The drawing under review shows one solid part. Ordinate dimensions are in mm from its lowest x, y, z. Round coordinates to 2 decimals unless told otherwise and drop trailing zeros. Order: outer loops, then holes, each group sorted by start corner. A loop starts at its lowest first (then second) coordinate and runs counter-clockwise, first axis right, second up. Notation, with made-up numbers: M -39.75,36 L 19.25,36 A12 ccw 19.25,48 Z; hole C -9,-5.5 d4. An arc over 180 degrees is marked long. Answer as a JSON object with one key per item and string values. Group by question number.
1. Clearance check with flat-ended pins moving along their axes: P1, Ø6, axis at x = 23, y = 5, coming from the -Z side; P2, Ø3.5, axis at x = 50, y = 12.5, coming from the -Z side. State where each tip first meets the part, or that it passes through.
2. To check wall thickness, follow probe 1 along Y at (x, z) = (50, 3.5); probe 2 along X at (y, z) = (12.5, 4.25); probe 3 along X at (y, z) = (13.25, 0.5). State the ranges of each line that lie inside material, in increasing order. Write a range as [from, to].
3. Add section B-B on y = 12.5. State the section outline as (x, z) points, and give its area (3 significant figures).
4. Add section A-A on x = 50. State the section outline as (y, z) points, and give its area (3 significant figures).
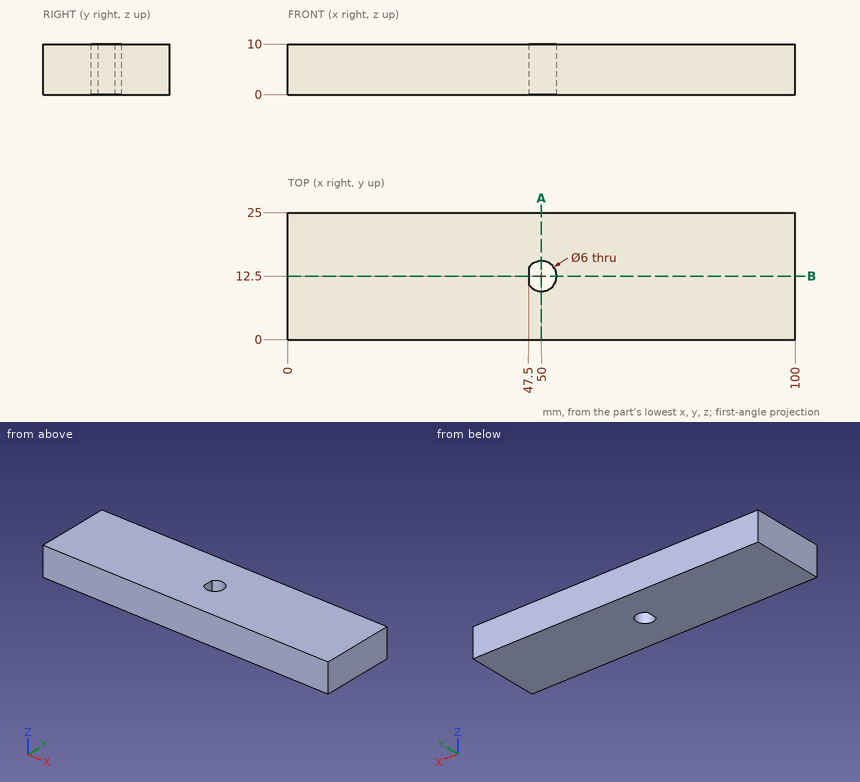
Recorded:
{
 "1": {"P1": "stops at z = 0", "P2": "passes through"},
 "2": {"probe 1": "y = [0, 9.5], [15.5, 25]", "probe 2": "x = [0, 47.5], [53, 100]", "probe 3": "x = [0, 47.5], [52.9, 100]"},
 "3": {"outline": "M 0,0 L 47.5,0 L 47.5,10 L 0,10 Z; M 53,0 L 100,0 L 100,10 L 53,10 Z", "area": "945 mm²"},
 "4": {"outline": "M 0,0 L 9.5,0 L 9.5,10 L 0,10 Z; M 15.5,0 L 25,0 L 25,10 L 15.5,10 Z", "area": "190 mm²"}
}
